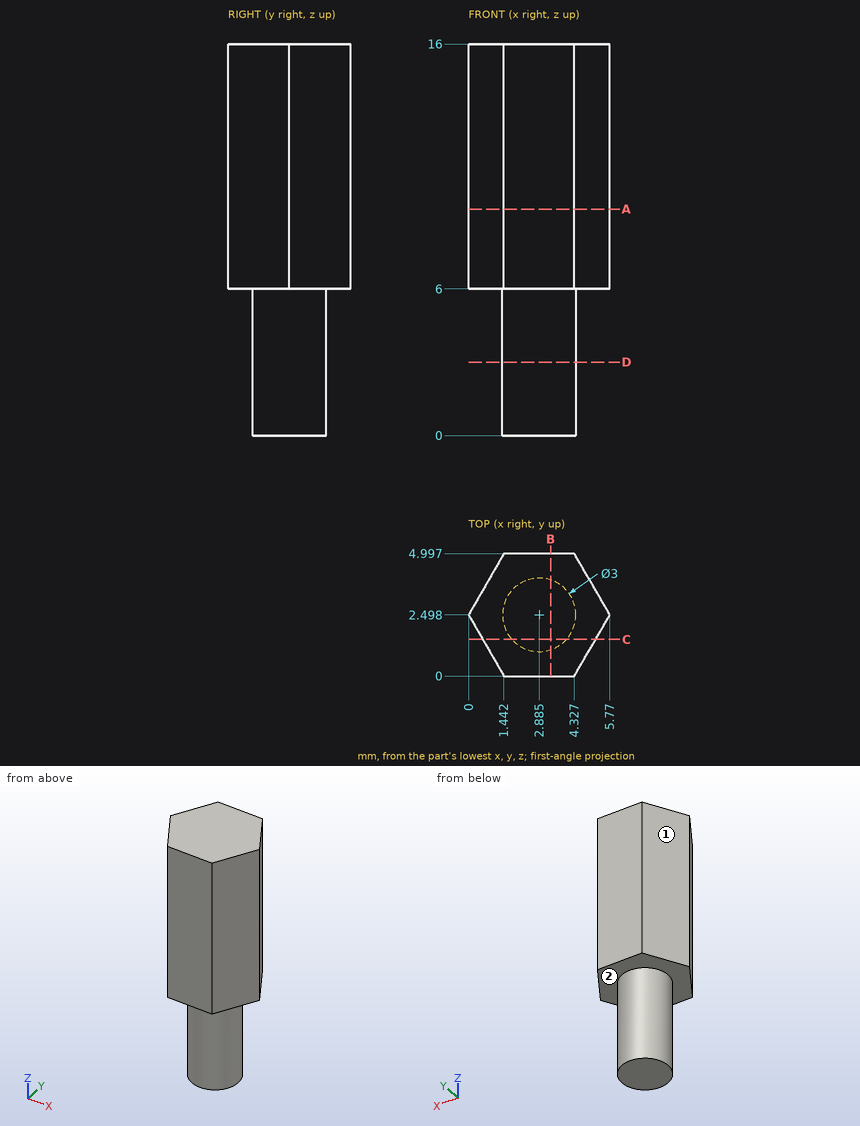
Could you check a few things on this drawing? It's one solid part, dimensions in mm from its lowest x, y, z. A direction names the side the tool comes from. Coordinates: 2 decimals unless noted, no trailing zeros. Order: outer loops, then holes, each group sorted by start corner. A loop starts at its lowest first (then second) coordinate and runs counter-clockwise, first axis right, second up.
1) Which directions (+Z, -Z, +X, -X, +Y, -Y) give clear straight access to the entire face, cutting with the end or side of a thin tool? Please do the marked faces 1 and 2.
2) Imagine slicing it at C-C on y = 1.5. List the corners of the cut face in (x, z) for me (1 decimal).
3) Imagine slicing it at B-B on x = 3.35. List the corners of the cut face in (y, z) for me (1 decimal).
4) Imagine slicing it at A-A on z = 9.25. List the corners of the cut face in (x, y) for me, and give its area (3 significant figures).
5) I need wall thicknesses on line 1 (Z direction, x = 4.4, y = 1.35); line 2 (X direction, y = 3.55, z = 15.25) (1 decimal); line 3 (X direction, y = 2, z = 2). Which ranges of each line are inside material? Lowest first, please.
6) Imagine slicing it at D-D on z = 3. List the corners of the cut face in (x, y) for me (1 decimal).
7) Will these pins go through, and if not, where does the flat tip stop? pin 1 (1 mm diameter, centred on x = 2.5, z = 11, fed in from -Y); pin 2 (1.5 mm diameter, centred on y = 4.5, z = 9.5, fed in from +X); pin 3 (1 mm diameter, centred on x = 5, z = 2, fed in from +Y).
Response values:
1. face 1: +Z, -Z, -X, +Y
1. face 2: -Z
2. outline: (0.6, 6) - (1.8, 6) - (1.8, 0) - (4, 0) - (4, 6) - (5.2, 6) - (5.2, 16) - (0.6, 16) - close
3. outline: (0, 6) - (1.1, 6) - (1.1, 0) - (3.9, 0) - (3.9, 6) - (5, 6) - (5, 16) - (0, 16) - close
4. outline: (0, 2.5) - (1.44, 0) - (4.33, 0) - (5.77, 2.5) - (4.33, 5) - (1.44, 5) - close
4. area: 21.6 mm2
5. line 1: z = 6 to 16
5. line 2: x = 0.6 to 5.2
5. line 3: x = 1.47 to 4.3
6. outline: circle Ø3 at (2.9, 2.5)
7. pin 1: stops at y = 0
7. pin 2: stops at x = 5.05
7. pin 3: passes through
